The model under review builds one solid part; all positions refer to its coordinate system, in mm. A direction names the side the tool comes from. Round coordinates to 2 decimals unless told otherwise and drop trailing zeros. Write each loop counter-clockwise with the first axis right and the second up, starting at its lowest first coordinate (ties: lowest second). Pieces come first, ordered by that corner, then holes. Notation, with made-up numbers: M 33.25,-25.5 L 70.25,-25.5 A17 ccw 70.25,-10.5 Z; hole C -35.5,-6.5 d5. An arc over 180 degrees is marked long. Write item = value, one per line. Start each with the question number.
Item 1: Tool access review of faces 3 (the flat face through (37.6, 12.5, -1.553)), 4 (the flat face through (69, 0, 3.247)): name each direction out of +Z, -Z, +X, -X, +Y, -Y from which nothing blocks a thin tool from reaching the whole face with its end or side.
Item 2: To check wall thickness, follow line 1 along Y through (x, z) = (-10.5, 0); line 2 along Z through (x, y) = (23.5, 1); line 3 along Z through (x, y) = (48.5, -7). State the ranges of each line that lie inside material, in increasing order.
Item 3: Take a section at B-B, the plane x = 95. Give the boundary of the cut face in (y, z).
Item 4: The part is to be moulded in two halves that separate along X. For faces 1 (the flat face through (38, 15.2, 2)), 2 (the flat face through (45, 0, 3.247)), say which applies: +X half, -X half, draft (parallel to the pull), parting line (faces both ways), or undercut.
Item 5: For pin 1 Ø10 at (x, y) = (79.5, -8) entering from -Z; pin 2 Ø1.2 at (x, y) = (87.5, -2.5) entering from -Z; pin 3 Ø2.5 at (x, y) = (44.5, 3) entering from -Z, all flat-tipped, find the tip position at first contact; note any pin that passes through.
Item 6: Take a section at A-A, the plane z = 0. Give the boundary of the cut face in (x, y), plus the area to 3 significant figures.
from build123d import *

# Parameters (mm, degrees)
EXTRUDE_1_DEPTH = 2
SKETCH_2_W      = 1.5
SKETCH_2_H      = 12
EXTRUDE_2_DEPTH = 1
SKETCH_3_W      = 89.86690944
SKETCH_3_H      = 19
EXTRUDE_3_DEPTH = 4
SCALE_1_SCALE   = 1.6


with BuildPart() as part:
    # 草图1 → 凸台-拉伸1 (new body)
    with BuildSketch(Plane.XY):
        with BuildLine():
            Line((0, 7.5), (71.36690944, 7.5))
            Line((71.36690944, 7.5), (71.36690944, 6.01680195))
            Line((71.36690944, 6.01680195), (78.36690944, 6.01680195))
            Line((78.36690944, 6.01680195), (78.36690944, 7.5))
            Line((78.36690944, 7.5), (80.36690944, 7.5))
            Line((80.36690944, 7.5), (80.36690944, -7.5))
            Line((80.36690944, -7.5), (78.36690944, -7.5))
            Line((78.36690944, -7.5), (78.36690944, -6.01680195))
            Line((78.36690944, -6.01680195), (71.36690944, -6.01680195))
            Line((71.36690944, -6.01680195), (71.36690944, -7.5))
            Line((71.36690944, -7.5), (0, -7.5))
            ThreePointArc((0, -7.5), (-6.151670717, 0), (0, 7.5))
        make_face()
    extrude(amount=EXTRUDE_1_DEPTH)

    # 草图2 → 凸台-拉伸2 (add)
    with BuildSketch(Plane.XY.offset(2)):
        with Locations((3, 0)):
            Rectangle(SKETCH_2_W, SKETCH_2_H)
        with Locations((6, 0)):
            Rectangle(SKETCH_2_W, SKETCH_2_H)
        with Locations((9, 0)):
            Rectangle(SKETCH_2_W, SKETCH_2_H)
        with Locations((12, 0)):
            Rectangle(SKETCH_2_W, SKETCH_2_H)
        with Locations((15, 0)):
            Rectangle(SKETCH_2_W, SKETCH_2_H)
        with Locations((18, 0)):
            Rectangle(SKETCH_2_W, SKETCH_2_H)
        with Locations((21, 0)):
            Rectangle(SKETCH_2_W, SKETCH_2_H)
        with Locations((24, 0)):
            Rectangle(SKETCH_2_W, SKETCH_2_H)
        with Locations((27, 0)):
            Rectangle(SKETCH_2_W, SKETCH_2_H)
        with Locations((30, 0)):
            Rectangle(SKETCH_2_W, SKETCH_2_H)
        with Locations((33, 0)):
            Rectangle(SKETCH_2_W, SKETCH_2_H)
        with Locations((36, 0)):
            Rectangle(SKETCH_2_W, SKETCH_2_H)
        with Locations((39, 0)):
            Rectangle(SKETCH_2_W, SKETCH_2_H)
        with Locations((42, 0)):
            Rectangle(SKETCH_2_W, SKETCH_2_H)
        with Locations((45, 0)):
            Rectangle(SKETCH_2_W, SKETCH_2_H)
        with Locations((48, 0)):
            Rectangle(SKETCH_2_W, SKETCH_2_H)
        with Locations((51, 0)):
            Rectangle(SKETCH_2_W, SKETCH_2_H)
        with Locations((54, 0)):
            Rectangle(SKETCH_2_W, SKETCH_2_H)
        with Locations((57, 0)):
            Rectangle(SKETCH_2_W, SKETCH_2_H)
        with Locations((60, 0)):
            Rectangle(SKETCH_2_W, SKETCH_2_H)
        with Locations((63, 0)):
            Rectangle(SKETCH_2_W, SKETCH_2_H)
        with Locations((66, 0)):
            Rectangle(SKETCH_2_W, SKETCH_2_H)
        with Locations((69, 0)):
            Rectangle(SKETCH_2_W, SKETCH_2_H)
    extrude(amount=EXTRUDE_2_DEPTH)


with BuildPart() as body_2:
    # 草图3 → 凸台-拉伸3 (new body)
    with BuildSketch(Plane(origin=(0, 0, 0), x_dir=(-1, 0, 0), z_dir=(0, 0, -1))):
        with Locations((-37.43345472, 0)):
            Rectangle(SKETCH_3_W, SKETCH_3_H)
    extrude(amount=-EXTRUDE_3_DEPTH)

    # Combine 1: cut part
    add(part.part, mode=Mode.SUBTRACT)


with BuildPart() as body_2_1:
    # 缩放比例1: scaled about (37.701981545, 0, 2.588708168)
    add(body_2.part.scale(SCALE_1_SCALE).moved(Location((-22.621188927, 0, -1.553224901))))


solid = body_2_1.part
Response values:
q1.face_3 = -Z, +X, -X, +Y, -Y
q1.face_4 = -Z
q2.line_1 = -15.2 to -12, 12 to 15.2
q2.line_2 = 1.65 to 4.85
q2.line_3 = 3.25 to 4.85
q3.outline = M -15.2,-1.55 L -9.63,-1.55 L -9.63,1.65 L 9.63,1.65 L 9.63,-1.55 L 15.2,-1.55 L 15.2,4.85 L -15.2,4.85 Z
q4.face_1 = draft
q4.face_2 = undercut
q5.pin_1 = -1.55
q5.pin_2 = 3.25
q5.pin_3 = 1.65
q6.outline = M -34.62,-15.2 L 109.17,-15.2 L 109.17,15.2 L -34.62,15.2 Z; hole M -22.62,-12 L 91.57,-12 L 91.57,-9.63 L 102.77,-9.63 L 102.77,-12 L 105.97,-12 L 105.97,12 L 102.77,12 L 102.77,9.63 L 91.57,9.63 L 91.57,12 L -22.62,12 A12.24 ccw Z
q6.area = 1,160 mm2
